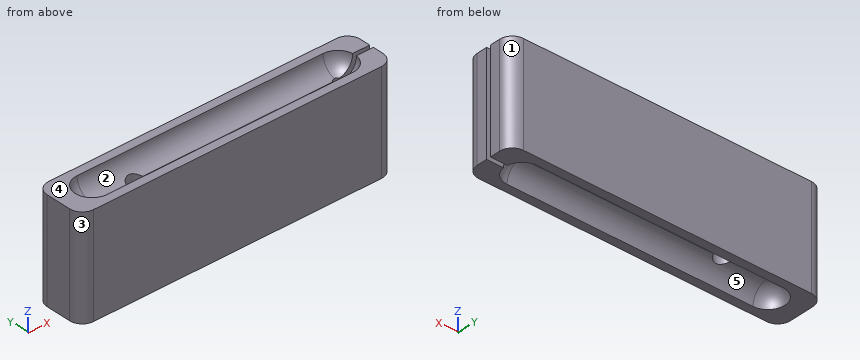
```python
from build123d import *

# Parameters (mm, degrees)
BOSS_EXTRUDE1_DEPTH = 76.2


with BuildPart() as part:
    # Sketch1 → Boss-Extrude1 (new body)
    with BuildSketch(Plane.XY):
        with BuildLine():
            Line((0, 20.6375), (0, 28.575))
            ThreePointArc((0, 28.575), (-2.789807909, 35.310192091), (-9.525, 38.1))
            Line((-9.525, 38.1), (-227.203, 38.1))
            ThreePointArc((-227.203, 38.1), (-233.938192091, 35.310192091), (-236.728, 28.575))
            Line((-236.728, 28.575), (-236.728, 9.525))
            ThreePointArc((-236.728, 9.525), (-233.938192091, 2.789807909), (-227.203, 0))
            Line((-227.203, 0), (-9.525, 0))
            ThreePointArc((-9.525, 0), (-2.789807909, 2.789807909), (0, 9.525))
            Line((0, 9.525), (0, 17.4625))
            Line((0, 17.4625), (-22.650369343, 17.4625))
            ThreePointArc((-22.650369343, 17.4625), (-25.4, 15.875), (-28.149630657, 17.4625))
            Line((-28.149630657, 17.4625), (-171.651638938, 17.4625))
            ThreePointArc((-171.651638938, 17.4625), (-184.15, 19.05), (-171.651638938, 20.6375))
            Line((-171.651638938, 20.6375), (-28.149630657, 20.6375))
            ThreePointArc((-28.149630657, 20.6375), (-25.4, 22.225), (-22.650369343, 20.6375))
            Line((-22.650369343, 20.6375), (0, 20.6375))
        make_face()
    extrude(amount=BOSS_EXTRUDE1_DEPTH)

    # Sketch2 → Cut-Revolve1 (revolve, cut)
    with BuildSketch(Plane.XY.offset(76.2)):
        with BuildLine():
            Line((-211.328, 31.75), (-25.4, 31.75))
            ThreePointArc((-25.4, 31.75), (-16.419743879, 28.030256121), (-12.7, 19.05))
            Line((-12.7, 19.05), (-224.028, 19.05))
            ThreePointArc((-224.028, 19.05), (-220.308256121, 28.030256121), (-211.328, 31.75))
        make_face()
    revolve(axis=Axis((-224.028, 19.05, 76.2), (1, 0, 0)), mode=Mode.SUBTRACT)

    # Sketch4 → Cut-Revolve3 (revolve, cut)
    with BuildSketch(Plane(origin=(0, 0, 0), x_dir=(-1, 0, 0), z_dir=(0, 0, -1))):
        with BuildLine():
            Line((25.4, 31.75), (211.328, 31.75))
            ThreePointArc((211.328, 31.75), (220.308256121, 28.030256121), (224.028, 19.05))
            Line((224.028, 19.05), (12.7, 19.05))
            ThreePointArc((12.7, 19.05), (16.419743879, 28.030256121), (25.4, 31.75))
        make_face()
    revolve(axis=Axis((-224.028, 19.05, 0), (1, 0, 0)), mode=Mode.SUBTRACT)


solid = part.part
```
Can you work these out from the model? Positions are in its coordinate system, mm. Face numbers are marked on the shaded views. A direction names the side the tool comes from. Coordinates: 2 decimals unless noted, no trailing zeros. Loops run counter-clockwise (first coordinate to the right, second up) from the corner with the lowest first, then second, coordinate; pieces in that order, holes last. Notation, with made-up numbers: (-10.5, 29) - (6.5, 29) arc R36 cw to (6.5, 68) - close; hole circle Ø8 at (-31.75, 35). An arc over 180 degrees is marked (long way). Use a Markdown table: item, result.
Item 1: I want a section at D-D on y = 3.5. Please give me the cut outline in (x, z).
Numbers:
| item | result |
|---|---|
| outline | (-234.58, 0) - (-2.15, 0) - (-2.15, 76.2) - (-234.58, 76.2) - close |
Item 2: For the marked faces 1 and 2, which set-ups out of +Z, -Z, +X, -X, +Y, -Y let a thin tool reach every point of the face, with its end or its side?
Numbers:
| item | result |
|---|---|
| face 1 | +Z, -Z, +X, +Y |
| face 2 | +Z |
Item 3: If I drill on probe 1 along Y at (x, z) = (-39.5, 48.5); probe 2 along Y at (x, z) = (-177.8, 45); probe 3 along X at (y, z) = (17, 60.5), over which ranges is the centre line in solid material (lowest first)? Write a range as from..to.
Numbers:
| item | result |
|---|---|
| probe 1 | y = 0..17.46, 20.64..38.1 |
| probe 2 | y = 0..12.7, 25.4..38.1 |
| probe 3 | x = -236.73..-183.81, -171.79..-27.82, -22.98..0 |
Item 4: I want a section at A-A on x = -177.8. Please give me the cut outline in (y, z).
Numbers:
| item | result |
|---|---|
| outline | (0, 0) - (6.35, 0) arc R12.7 cw to (12.7, 11) - (12.7, 65.2) arc R12.7 cw to (6.35, 76.2) - (0, 76.2) - close; (25.4, 11) arc R12.7 cw to (31.75, 0) - (38.1, 0) - (38.1, 76.2) - (31.75, 76.2) arc R12.7 cw to (25.4, 65.2) - close |
Item 5: I want a section at C-C on x = -202. Please give me the cut outline in (y, z).
Numbers:
| item | result |
|---|---|
| outline | (0, 0) - (6.35, 0) arc R12.7 cw to (31.75, 0) - (38.1, 0) - (38.1, 76.2) - (31.75, 76.2) arc R12.7 cw to (6.35, 76.2) - (0, 76.2) - close |
Item 6: We'd pull the mould along Y, two halves only. Please class the marked faces 3, 4 and 5: released by +Y, released by -Y, zero draft, split by the parting line, or undercut.
Numbers:
| item | result |
|---|---|
| face 3 | released by -Y |
| face 4 | zero draft |
| face 5 | undercut |
Item 7: Will these pins go through, and if not, where does the flat tip stop? pin 1 (4 mm diameter, centred on x = -141, y = 23.5, fed in from -Z); pin 2 (20.5 mm diameter, centred on x = -177.8, y = 19.05, fed in from -Z); pin 3 (2 mm diameter, centred on y = 4.5, z = 8.5, fed in from +X).
Numbers:
| item | result |
|---|---|
| pin 1 | stops at z = 10.94 |
| pin 2 | stops at z = 7.5 |
| pin 3 | stops at x = -0.89 |
